For this review, take the finished solid that the model builds, in its own axes (mm). A direction names the side the tool comes from. Round coordinates to 2 decimals unless told otherwise and drop trailing zeros. Write each loop counter-clockwise with the first axis right and the second up, starting at its lowest first coordinate (ties: lowest second). Pieces come first, ordered by that corner, then holes. Notation, with made-up numbers: (9.5, -8.75) -> (45.5, -8.75) arc R31 ccw to (45.5, 22.25) -> close; hole circle Ø1 at (1.5, 1.25). An arc over 180 degrees is marked (long way). Answer in a Markdown table with one row per item. Add a question column.
```python
from build123d import *

# Parameters (mm, degrees)
EXTRUDE_1_DEPTH     = 14.15
SKETCH_2_W          = 30.4
SKETCH_2_H          = 30.4
CUT_EXTRUDE_1_DEPTH = 11.35
CUT_EXTRUDE_2_REACH = 53.48
CUT_EXTRUDE_3_REACH = 53.48


with BuildPart() as part:
    # 草图1 → 凸台-拉伸1 (new, symmetric)
    with BuildSketch(Plane.XY):
        Polygon((0, 0), (35, 0), (35, 35), (29, 35), (29, 29), (6, 6), (0, 6), align=None)
    extrude(amount=EXTRUDE_1_DEPTH, both=True)

    # 草图2 → 切除-拉伸1 (cut, symmetric)
    with BuildSketch(Plane.XY):
        with Locations((15.2, 19.8)):
            Rectangle(SKETCH_2_W, SKETCH_2_H)
    extrude(amount=CUT_EXTRUDE_1_DEPTH, both=True, mode=Mode.SUBTRACT)

    # 草图4 → 切除-拉伸2 (cut, up to next)
    with BuildSketch(Plane(origin=(0, 0, 0), x_dir=(1, 0, 0), z_dir=(0, 1, 0)), mode=Mode.PRIVATE) as cut_extrude_2_sk1:
        with BuildLine():
            Line((10.85, 3.25), (24.15, 3.25))
            ThreePointArc((24.15, 3.25), (27.4, 0), (24.15, -3.25))
            Line((24.15, -3.25), (10.85, -3.25))
            ThreePointArc((10.85, -3.25), (7.6, 0), (10.85, 3.25))
        make_face()
    cut_extrude_2_tool1 = extrude(cut_extrude_2_sk1.sketch, amount=CUT_EXTRUDE_2_REACH, mode=Mode.PRIVATE) & part.part
    add(cut_extrude_2_tool1.solids().sort_by_distance((17.5, 0, 0))[0], mode=Mode.SUBTRACT)

    # 草图5 → 切除-拉伸3 (cut, up to next)
    with BuildSketch(Plane(origin=(0, 0, 0), x_dir=(0, 0, -1), z_dir=(1, 0, 0)), mode=Mode.PRIVATE) as cut_extrude_3_sk1:
        with BuildLine():
            Line((-3.25, 10.85), (-3.25, 24.15))
            ThreePointArc((-3.25, 24.15), (0, 27.4), (3.25, 24.15))
            Line((3.25, 24.15), (3.25, 10.85))
            ThreePointArc((3.25, 10.85), (0, 7.6), (-3.25, 10.85))
        make_face()
    cut_extrude_3_tool1 = extrude(cut_extrude_3_sk1.sketch, amount=CUT_EXTRUDE_3_REACH, mode=Mode.PRIVATE) & part.part
    add(cut_extrude_3_tool1.solids().sort_by_distance((0, 17.5, 0))[0], mode=Mode.SUBTRACT)


solid = part.part
```
1. We need section A-A (y = 18.5). Write out the cut boundary in (x, z), plus the area to 3 significant figures.
2. Clearance check with flat-ended pins moving along their axes: pin 1 Ø0.8 at (y, z) = (31, 12.5) entering from -X; pin 2 Ø1.4 at (x, z) = (3.5, 13) entering from +Y; pin 3 Ø5 at (y, z) = (8.5, 5) entering from -X. State where each tip first meets the part, or that it passes through.
3. The part is to be moulded in two halves that separate along Y. For faces 5 (the flat face through (18, 2, 3.25)), 6 (the flat face through (33, 17, 3.25)), 7 (the flat face through (17, 0, 6)), say which applies: pulls with the +Y half, pulls with the -Y half, needs draft (parallel to the pull), parting line crosses it, or undercut.
4. We need section D-D (x = 14.5). Write out the cut boundary in (y, z).
5. We need section B-B (x = 32). Write out the cut boundary in (y, z).
6. We need section C-C (z = 0.25). Write out the cut boundary in (x, y).
7. Tool access review of faces 1 (the flat face through (22, 13, 11.35)), 2 (the flat face through (29, 32, -13)), 3 (the flat face through (33, 18, -3.25)), 4 (the cylindrical face through (7.6, 2.3, 0.1)): name each direction out of +Z, -Z, +X, -X, +Y, -Y from which nothing blocks a thin tool from reaching the whole face with its end or side.
8. For L1, parallel to Z at x = 25.5, y = 21; L2, parallel to Z at x = 15, y = 2.5; L3, parallel to X at y = 8, z = -6, list the stretches that pass through material, from the lowest coordinate up. Write a range as [from, to].
Response:
| question | item | result |
|---|---|---|
| 1 | outline | (18.5, -14.15) -> (35, -14.15) -> (35, -3.25) -> (30.4, -3.25) -> (30.4, -11.35) -> (18.5, -11.35) -> close; (18.5, 11.35) -> (30.4, 11.35) -> (30.4, 3.25) -> (35, 3.25) -> (35, 14.15) -> (18.5, 14.15) -> close |
| 1 | area | 167 mm2 |
| 2 | pin 1 | x = 29 |
| 2 | pin 2 | y = 6 |
| 2 | pin 3 | x = 30.4 |
| 3 | face 5 | needs draft |
| 3 | face 6 | undercut |
| 3 | face 7 | pulls with the -Y half |
| 4 | outline | (0, -14.15) -> (14.5, -14.15) -> (14.5, -11.35) -> (4.6, -11.35) -> (4.6, -3.25) -> (0, -3.25) -> close; (0, 3.25) -> (4.6, 3.25) -> (4.6, 11.35) -> (14.5, 11.35) -> (14.5, 14.15) -> (0, 14.15) -> close |
| 5 | outline | (0, -14.15) -> (35, -14.15) -> (35, 14.15) -> (0, 14.15) -> close; hole (10.85, -3.25) -> (24.15, -3.25) arc R3.25 ccw to (24.15, 3.25) -> (10.85, 3.25) arc R3.25 ccw to start |
| 6 | outline | (0, 0) -> (7.61, 0) -> (7.61, 4.6) -> (0, 4.6) -> close; (27.39, 0) -> (35, 0) -> (35, 7.61) -> (30.4, 7.61) -> (30.4, 4.6) -> (27.39, 4.6) -> close; (30.4, 27.39) -> (35, 27.39) -> (35, 35) -> (30.4, 35) -> close |
| 7 | face 1 | -X, +Y |
| 7 | face 2 | +Z, -Z, -X, +Y |
| 7 | face 3 | +X, -X |
| 7 | face 4 | +Y, -Y |
| 8 | L1 | [-14.15, -11.35], [11.35, 14.15] |
| 8 | L2 | [-14.15, -3.25], [3.25, 14.15] |
| 8 | L3 | [30.4, 35] |
